Read the model definition and answer for the solid it produces. Units are mm, in the model's axes. Face numbers are marked on the shaded views. A direction names the side the tool comes from. Coordinates: 2 decimals unless noted, no trailing zeros. Write each loop counter-clockwise with the first axis right and the second up, starting at its lowest first coordinate (ties: lowest second). Pieces come first, ordered by that corner, then holes. Notation, with made-up numbers: (-36.75, 48.25) -> (3.25, 48.25) arc R27 ccw to (3.25, 84.25) -> close; hole circle Ø5 at (-27.75, -40). An arc over 180 degrees is marked (long way). Answer in a Markdown table with one row per item. Add a question column.
Item 1: Which of the six approach directions +Z, -Z, +X, -X, +Y, -Y give full straight-line access (tool end or side, diameter ignored) to the marked faces 1 and 2?
Item 2: Section B-B on x = 27 is taken. Write down the section's boundary in (y, z), then the cut area to 3 significant figures.
Item 3: Section A-A on y = 365 is taken. Write down the section's boundary in (x, z).
Item 4: Section C-C on x = 0 is taken. Write down the section's boundary in (y, z), then the cut area to 3 significant figures.
Item 5: Straight lines are drawn through the part: line 1 (Y direction, x = 0, z = 46); line 2 (Z direction, x = 22.5, y = 344); line 3 (Z direction, x = -14, y = 80.5). For each, find the intervals that lie inside material, in ascending order. Write a range as from..to.
Item 6: For a pull along Z with two mould halves and no side action, classify the marked faces 3, 4, 5 and 6 as +Z half, -Z half, draft (parallel to the pull), parting line (faces both ways), or undercut.
Item 7: Given pin 1 Ø5 at (y, z) = (349, -34) entering from +X; pin 2 Ø8 at (x, y) = (8.5, 314) entering from +Z; pin 3 Ø8 at (x, y) = (31.5, 224.5) entering from -Z; pin 4 Ø1 at (x, z) = (-39.5, 37.5) entering from -Y, each flat-ended and moving along its own axis, determine where each tip first touches the part or whether it passes through.
Item 8: Section D-D on y = 40 is taken. Write down the section's boundary in (x, z), then the cut area to 3 significant figures.
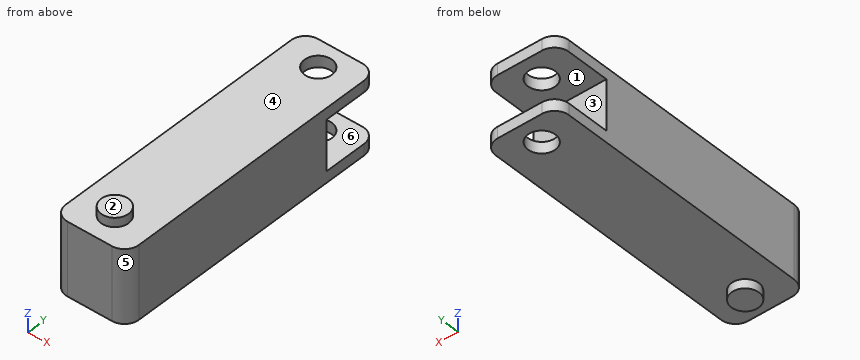
```python
from build123d import *

# Parameters (mm, degrees)
CROQUIS1_W              = 101.6
CROQUIS1_H              = 101.6
SALIENTE_EXTRUIR1_DEPTH = 400
CROQUIS2_R              = 19.05
SALIENTE_EXTRUIR2_DEPTH = 12.7
SALIENTE_EXTRUIR3_START = 12.7
CROQUIS3_R              = 19.05
SALIENTE_EXTRUIR3_DEPTH = 12.7
REDONDEO1_R             = 20
CROQUIS5_W              = 70
CROQUIS5_H              = 80
CORTAR_EXTRUIR1_DEPTH   = 101.6
CORTAR_EXTRUIR2_REACH   = 421.1
CROQUIS6_R              = 19.05
REDONDEO2_R             = 20


with BuildPart() as part:
    # Croquis1 → Saliente-Extruir1 (new body)
    with BuildSketch(Plane(origin=(0, 0, 0), x_dir=(1, 0, 0), z_dir=(0, 1, 0))):
        Rectangle(CROQUIS1_W, CROQUIS1_H)
    extrude(amount=SALIENTE_EXTRUIR1_DEPTH)

    # Croquis2 → Saliente-Extruir2 (add)
    with BuildSketch(Plane.XY.offset(50.8)):
        with Locations(Location((0, 40, 0), (0, 0, 180))):
            Circle(CROQUIS2_R)
    extrude(amount=SALIENTE_EXTRUIR2_DEPTH)

    # Croquis3 → Saliente-Extruir3 (add)
    with BuildSketch(Plane(origin=(0, 0, -50.8), x_dir=(-1, 0, 0), z_dir=(0, 0, -1)).offset(SALIENTE_EXTRUIR3_START)):
        with Locations((0, 40)):
            Circle(CROQUIS3_R)
    extrude(amount=-SALIENTE_EXTRUIR3_DEPTH)

    # Redondeo1
    redondeo1_edges = [part.edges().sort_by_distance(p)[0] for p in [
        (-50.8, 0, 0),
        (50.8, 0, 0),
    ]]
    fillet(redondeo1_edges, radius=REDONDEO1_R)

    # Croquis5 → Cortar-Extruir1 (cut)
    with BuildSketch(Plane(origin=(50.8, 0, 0), x_dir=(0, 0, -1), z_dir=(1, 0, 0))):
        with Locations((0, 360)):
            Rectangle(CROQUIS5_W, CROQUIS5_H)
    extrude(amount=-CORTAR_EXTRUIR1_DEPTH, mode=Mode.SUBTRACT)

    # Cortar-Extruir2: up to this face of the body (flat: up to its plane)
    cortar_extruir2_end = Plane(part.part.faces().sort_by_distance((0, 205.491832247, 50.8))[0])
    # Croquis6 → Cortar-Extruir2 (cut, up to the picked face)
    with BuildSketch(Plane(origin=(0, 0, -50.8), x_dir=(-1, 0, 0), z_dir=(0, 0, -1)), mode=Mode.PRIVATE) as cortar_extruir2_sk1:
        with Locations((0, 365)):
            Circle(CROQUIS6_R)
    cortar_extruir2_tool1 = split(extrude(cortar_extruir2_sk1.sketch, amount=-CORTAR_EXTRUIR2_REACH, mode=Mode.PRIVATE), bisect_by=cortar_extruir2_end, keep=Keep.BOTH, mode=Mode.PRIVATE)
    add(cortar_extruir2_tool1.solids().sort_by(Axis((0, 365, -50.8), (0, 0, 1)))[0], mode=Mode.SUBTRACT)

    # Redondeo2
    redondeo2_edges = [part.edges().sort_by_distance(p)[0] for p in [
        (-50.8, 400, -42.9),
        (50.8, 400, -42.9),
        (-50.8, 400, 42.9),
        (50.8, 400, 42.9),
    ]]
    fillet(redondeo2_edges, radius=REDONDEO2_R)


solid = part.part
```
Results below:
| question | item | result |
|---|---|---|
| 1 | face 1 | +X, -X, +Y |
| 1 | face 2 | +Z, +X, -X, +Y, -Y |
| 2 | outline | (0, -50.8) -> (400, -50.8) -> (400, -35) -> (320, -35) -> (320, 35) -> (400, 35) -> (400, 50.8) -> (0, 50.8) -> close |
| 2 | area | 35,000 mm2 |
| 3 | outline | (-50.8, -50.8) -> (-19.05, -50.8) -> (-19.05, -35) -> (-50.8, -35) -> close; (-50.8, 35) -> (-19.05, 35) -> (-19.05, 50.8) -> (-50.8, 50.8) -> close; (19.05, -50.8) -> (50.8, -50.8) -> (50.8, -35) -> (19.05, -35) -> close; (19.05, 35) -> (50.8, 35) -> (50.8, 50.8) -> (19.05, 50.8) -> close |
| 4 | outline | (0, -50.8) -> (20.95, -50.8) -> (20.95, -63.5) -> (59.05, -63.5) -> (59.05, -50.8) -> (345.95, -50.8) -> (345.95, -35) -> (320, -35) -> (320, 35) -> (345.95, 35) -> (345.95, 50.8) -> (59.05, 50.8) -> (59.05, 63.5) -> (20.95, 63.5) -> (20.95, 50.8) -> (0, 50.8) -> close; (384.05, -50.8) -> (400, -50.8) -> (400, -35) -> (384.05, -35) -> close; (384.05, 35) -> (400, 35) -> (400, 50.8) -> (384.05, 50.8) -> close |
| 4 | area | 34,800 mm2 |
| 5 | line 1 | y = 0..345.95, 384.05..400 |
| 5 | line 2 | z = -50.8..-35, 35..50.8 |
| 5 | line 3 | z = -50.8..50.8 |
| 6 | face 3 | undercut |
| 6 | face 4 | +Z half |
| 6 | face 5 | draft |
| 6 | face 6 | undercut |
| 7 | pin 1 | stops at x = 50.8 |
| 7 | pin 2 | stops at z = 50.8 |
| 7 | pin 3 | stops at z = -50.8 |
| 7 | pin 4 | stops at y = 1.76 |
| 8 | outline | (-50.8, -50.8) -> (-19.05, -50.8) -> (-19.05, -63.5) -> (19.05, -63.5) -> (19.05, -50.8) -> (50.8, -50.8) -> (50.8, 50.8) -> (19.05, 50.8) -> (19.05, 63.5) -> (-19.05, 63.5) -> (-19.05, 50.8) -> (-50.8, 50.8) -> close |
| 8 | area | 11,300 mm2 |
